Here's how the part is built. I have some questions about the finished solid (model axes, mm). Coordinates: 2 decimals unless noted, no trailing zeros. Write each loop counter-clockwise with the first axis right and the second up, starting at its lowest first coordinate (ties: lowest second). Pieces come first, ordered by that corner, then holes.
(1) For pin 1 Ø2.5 at (x, y) = (109.35, 111.125) entering from -Z; pin 2 Ø0.8 at (x, y) = (98.5, 71) entering from +Z, each with a flat end and sliding along its axis, tell me the tip position at first contact or that it passes through.
(2) Imagine slicing it at C-C, the plane x = 109.35. List the corners of the cut face in (y, z) for me.
(3) Imagine slicing it at D-D, the plane y = 107. List the corners of the cut face in (x, z) for me (3 decimals).
(4) Please list where these lines run through material, in increasing order: probe 1 along X at (y, z) = (101.6, -1.95); probe 2 along Y at (x, z) = (95.25, -0.85); probe 3 along X at (y, z) = (116.5, -0.5).
(5) Imagine slicing it at A-A, the plane x = 101.6. State how many separate pieces and enclosed holes the cut face has, plus the area to 3 significant figures.
(6) Imagine slicing it at B-B, the plane y = 82.55. List the corners of the cut face in (x, z) for me (1 decimal), plus the area to 3 significant figures.
```python
from build123d import *

# Parameters (mm, degrees)
EXTRUDE1_DEPTH     = 2.54
SKETCH2_R          = 1.5875
CUT_EXTRUDE1_DEPTH = 2.54
SKETCH3_W          = 2.794
SKETCH3_H          = 8.128
CUT_EXTRUDE2_DEPTH = 0.381
SKETCH4_R          = 0.7112
CUT_EXTRUDE3_DEPTH = 53.34
FILLET1_R          = 3.81
SKETCH5_R          = 1.5875
CUT_EXTRUDE4_DEPTH = 2.54


with BuildPart() as part:
    # Sketch1 → Extrude1 (new body)
    with BuildSketch(Plane.XY):
        Polygon((88.9, 127), (88.9, 63.5), (95.25, 25.4), (107.95, 25.4), (114.3, 63.5), (114.3, 127), align=None)
    extrude(amount=-EXTRUDE1_DEPTH)

    # Sketch2 → Cut-Extrude1 (cut)
    with BuildSketch(Plane.XY):
        with Locations((93.850000001, 111.125)):
            Circle(SKETCH2_R)
        with Locations((101.6, 120.65)):
            Circle(SKETCH2_R)
        with Locations((109.349999999, 111.125)):
            Circle(SKETCH2_R)
        with Locations((101.6, 101.6)):
            Circle(SKETCH2_R)
        with Locations((93.850000001, 92.075)):
            Circle(SKETCH2_R)
        with Locations((109.349999999, 92.075)):
            Circle(SKETCH2_R)
        with Locations((101.6, 82.55)):
            Circle(SKETCH2_R)
    extrude(amount=-CUT_EXTRUDE1_DEPTH, mode=Mode.SUBTRACT)

    # Sketch3 → Cut-Extrude2 (cut)
    with BuildSketch(Plane.XY):
        with Locations((97.725, 71.374)):
            Rectangle(SKETCH3_W, SKETCH3_H)
        with Locations((105.475, 71.374)):
            Rectangle(SKETCH3_W, SKETCH3_H)
    extrude(amount=-CUT_EXTRUDE2_DEPTH, mode=Mode.SUBTRACT)

    # Sketch4 → Cut-Extrude3 (cut)
    with BuildSketch(Plane(origin=(0, 127, 0), x_dir=(1, 0, 0), z_dir=(0, 1, 0))):
        with Locations((97.725, 0)):
            Circle(SKETCH4_R)
        with Locations((105.475, 0)):
            Circle(SKETCH4_R)
    extrude(amount=-CUT_EXTRUDE3_DEPTH, mode=Mode.SUBTRACT)

    # Fillet1
    fillet1_edges = [part.edges().sort_by_distance(p)[0] for p in [
        (95.25, 25.4, -1.27),
        (88.9, 63.5, -1.27),
        (88.9, 127, -1.27),
        (114.3, 127, -1.27),
        (114.3, 63.5, -1.27),
        (107.95, 25.4, -1.27),
    ]]
    fillet(fillet1_edges, radius=FILLET1_R)

    # Sketch5 → Cut-Extrude4 (cut)
    with BuildSketch(Plane.XY):
        with Locations((101.6, 33.3375)):
            Circle(SKETCH5_R)
    extrude(amount=-CUT_EXTRUDE4_DEPTH, mode=Mode.SUBTRACT)


solid = part.part
```
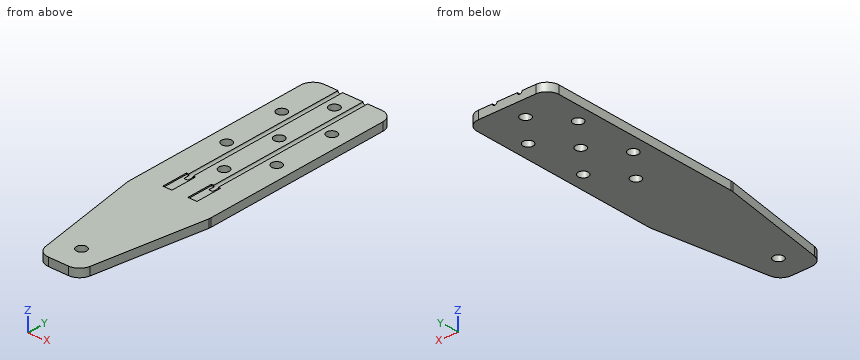
Recorded:
1. pin 1: passes through
1. pin 2: stops at z = -0.38
2. outline: (33.8, -2.54) - (90.49, -2.54) - (90.49, 0) - (33.8, 0) - close; (93.66, -2.54) - (109.54, -2.54) - (109.54, 0) - (93.66, 0) - close; (112.71, -2.54) - (127, -2.54) - (127, 0) - (112.71, 0) - close
3. outline: (88.9, -2.54) - (114.3, -2.54) - (114.3, 0) - (106.186, 0) arc R0.711 cw to (104.764, 0) - (98.436, 0) arc R0.711 cw to (97.014, 0) - (88.9, 0) - close
4. probe 1: x = 88.9 to 100.01, 103.19 to 114.3
4. probe 2: y = 27.19 to 91.33, 92.82 to 110.38, 111.87 to 127
4. probe 3: x = 88.9 to 97.22, 98.23 to 104.97, 105.98 to 114.3
5. separate pieces: 5
5. enclosed holes: 0
5. area: 226 mm2
6. outline: (88.9, -2.5) - (100, -2.5) - (100, 0) - (98.4, 0) arc R0.7 cw to (97, 0) - (88.9, 0) - close; (103.2, -2.5) - (114.3, -2.5) - (114.3, 0) - (106.2, 0) arc R0.7 cw to (104.8, 0) - (103.2, 0) - close
6. area: 54.9 mm2
